from build123d import *

# Parameters (mm, degrees)
F0_W     = 100
F0_H     = 100
F1_DEPTH = 100
F2_W     = 100
F2_H     = 80
F3_DEPTH = 40
F4_W     = 60
F4_H     = 40
F5_DEPTH = 100.001
F6_W     = 50
F6_H     = 40
F7_DEPTH = 100.001


with BuildPart() as f1:
    # F0 (on Top) → F1 (new body)
    with BuildSketch(Plane.XY):
        Rectangle(F0_W, F0_H)
    extrude(amount=F1_DEPTH)

    # F2 (on face) → F3 (cut)
    with BuildSketch(Plane.XY.offset(100)):
        with Locations((0, -10)):
            Rectangle(F2_W, F2_H)
    extrude(amount=-F3_DEPTH, mode=Mode.SUBTRACT)

    # F4 (on face) → F5 (cut, through all)
    with BuildSketch(Plane.XZ.offset(50)):
        with Locations((0, 20)):
            Rectangle(F4_W, F4_H)
    extrude(amount=-F5_DEPTH, mode=Mode.SUBTRACT)

    # F6 (on face) → F7 (cut, through all)
    with BuildSketch(Plane.YZ.offset(50)):
        with Locations((0, 20)):
            Rectangle(F6_W, F6_H)
    extrude(amount=-F7_DEPTH, mode=Mode.SUBTRACT)


solid = f1.part
The model under review builds one solid part; all positions refer to its coordinate system, in mm. A direction names the side the tool comes from. Give positions to 0.01 mm unless a question says otherwise; leave off trailing zeros. Loops run counter-clockwise (first coordinate to the right, second up) from the corner with the lowest first, then second, coordinate; pieces in that order, holes last. Notation, with made-up numbers: (40.5, -21) -> (82.5, -21) arc R11 cw to (82.5, -7) -> close; hole circle Ø7 at (-16.75, 29). An arc over 180 degrees is marked (long way). Put each result on its own line as item: value. Start each with the question number.
1. Clearance check with flat-ended pins moving along their axes: P1, Ø1.5, axis at x = 8, y = -23, coming from the +Z side; P2, Ø2, axis at x = 8, y = -28.5, coming from the -Z side; P3, Ø12, axis at x = -22, z = 84, coming from the -Y side. State where each tip first meets the part, or that it passes through.
2. Wall thickness on probe 1 along Y at (x, z) = (-34, 36); probe 2 along X at (y, z) = (42, 26.5); probe 3 along Z at (x, y) = (23, -32): over which ranges is each line inside the solid? List them lowest first.
3. Mouldability with a two-part tool opening along Y and no side actions: class faces 5 (the face through (40, -37, 0)), 6 (the face through (40, -25, 20)), 7 (the face through (-40, -25, 20)), 8 (the face through (-1, 30, 80)) as released by +Y, released by -Y, zero draft, split by the parting line, or undercut.
4. We need section A-A on z = 14. State the section outline as (x, y) points.
5. We need section B-B on y = -38.5. State the section outline as (x, z) points.
6. We need section C-C on x = -1. State the section outline as (y, z) points, then the cut area to 3 significant figures.
7. We need section D-D on z = 82. State the section outline as (x, y) points.
8. For faces 1 (the face through (30, -38, 20)), 2 (the face through (-1, -9, 60)), 3 (the face through (-40, -37, 0)), 4 (the face through (40, 25, 20)), list the 3-axis set-ups (+Z, -Z, +X, -X, +Y, -Y) from which the entire face can be reached by the end or side of a thin tool; tool diameter is ignored.
Determined:
1. P1: z = 60
1. P2: z = 40
1. P3: y = 30
2. probe 1: -50 to -25, 25 to 50
2. probe 2: -50 to -30, 30 to 50
2. probe 3: 40 to 60
3. face 5: zero draft
3. face 6: undercut
3. face 7: undercut
3. face 8: released by -Y
4. outline: (-50, -50) -> (-30, -50) -> (-30, -25) -> (-50, -25) -> close; (-50, 25) -> (-30, 25) -> (-30, 50) -> (-50, 50) -> close; (30, -50) -> (50, -50) -> (50, -25) -> (30, -25) -> close; (30, 25) -> (50, 25) -> (50, 50) -> (30, 50) -> close
5. outline: (-50, 0) -> (-30, 0) -> (-30, 40) -> (30, 40) -> (30, 0) -> (50, 0) -> (50, 60) -> (-50, 60) -> close
6. outline: (-50, 40) -> (50, 40) -> (50, 100) -> (30, 100) -> (30, 60) -> (-50, 60) -> close
6. area: 2,800 mm^2
7. outline: (-50, 30) -> (50, 30) -> (50, 50) -> (-50, 50) -> close
8. face 1: -Z, +Y, -Y
8. face 2: +Z, +X, -X, -Y
8. face 3: -Z, +X, -X, +Y, -Y
8. face 4: -Z, +X, -X
